For this review, take the finished solid that the model builds, in its own axes (mm). Face numbers are marked on the shaded views. A direction names the side the tool comes from. Coordinates: 2 decimals unless noted, no trailing zeros. Loops run counter-clockwise (first coordinate to the right, second up) from the corner with the lowest first, then second, coordinate; pieces in that order, holes last. Notation, with made-up numbers: (-0.5, 31.25) -> (49.5, 31.25) arc R20 cw to (49.5, 53.25) -> close; hole circle Ø11 at (-6, 89). An arc over 180 degrees is marked (long way). One line per item, written item: value.
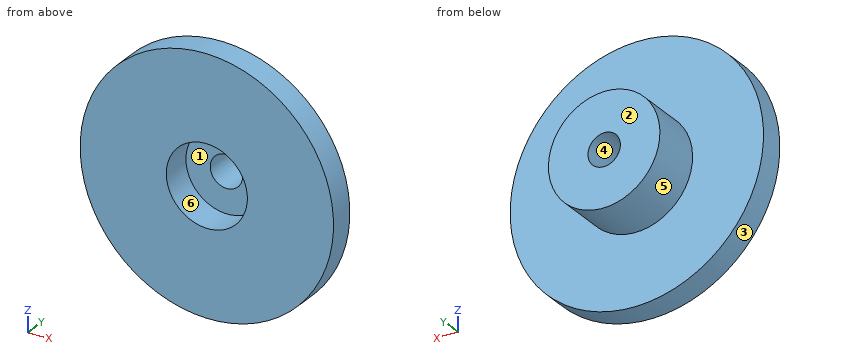
from build123d import *

# Parameters (mm, degrees)
SKETCH1_R           = 12.5
BOSS_EXTRUDE1_DEPTH = 2.5
SKETCH2_R           = 5.5
BOSS_EXTRUDE2_DEPTH = 5
HOLE1_D             = 3.2
HOLE1_DEPTH         = 100
HOLE1_CBORE_D       = 8
HOLE1_CBORE_DEPTH   = 3


with BuildPart() as part:
    # Sketch1 → Boss-Extrude1 (new body)
    with BuildSketch(Plane(origin=(0, 0, 0), x_dir=(1, 0, 0), z_dir=(0, 1, 0))):
        with Locations(Location((0, 0, 0), (0, 0, 270))):
            Circle(SKETCH1_R)
    extrude(amount=BOSS_EXTRUDE1_DEPTH)

    # Sketch2 → Boss-Extrude2 (add)
    with BuildSketch(Plane(origin=(0, 2.5, 0), x_dir=(1, 0, 0), z_dir=(0, 1, 0))):
        with Locations(Location((0, 0, 0), (0, 0, 270))):
            Circle(SKETCH2_R)
    extrude(amount=BOSS_EXTRUDE2_DEPTH)

    # Hole1
    with Locations(Plane(origin=(0, 0, 0), x_dir=(-1, 0, 0), z_dir=(0, -1, 0))):
        with Locations((0, 0)):
            CounterBoreHole(HOLE1_D / 2, HOLE1_CBORE_D / 2, HOLE1_CBORE_DEPTH, depth=HOLE1_DEPTH)


solid = part.part
1. For the marked faces 4, 5 and 6, list the 3-axis set-ups (+Z, -Z, +X, -X, +Y, -Y) from which the entire face can be reached by the end or side of a thin tool; tool diameter is ignored.
Return value:
face 4: +Y, -Y
face 5: +Y
face 6: -Y
2. To check wall thickness, follow probe 1 along X at (y, z) = (5.25, -0.25); probe 2 along Y at (x, z) = (-4.5, -9.5); probe 3 along Z at (x, y) = (1, 7.25). State the ranges of each line that lie inside material, in increasing order. Write a range as from..to.
Return value:
probe 1: x = -5.49..-1.58, 1.58..5.49
probe 2: y = 0..2.5
probe 3: z = -5.41..-1.25, 1.25..5.41
3. Take a section at C-C, the plane y = 4.5. Give the boundary of the cut face in (x, z), and give its area (3 significant figures).
Return value:
outline: circle Ø11 at (0, 0); hole circle Ø3.2 at (0, 0)
area: 87.0 mm2
4. Take a section at A-A, the plane z = 0. Give the boundary of the cut face in (x, y), and give its area (3 significant figures).
Return value:
outline: (-12.5, 0) -> (-4, 0) -> (-4, 3) -> (-1.6, 3) -> (-1.6, 7.5) -> (-5.5, 7.5) -> (-5.5, 2.5) -> (-12.5, 2.5) -> close; (1.6, 3) -> (4, 3) -> (4, 0) -> (12.5, 0) -> (12.5, 2.5) -> (5.5, 2.5) -> (5.5, 7.5) -> (1.6, 7.5) -> close
area: 79.1 mm2
5. The part is to be moulded in two halves that separate along X. For the marked faces 1, 2 and 3, say which applies: pulls with the +X half, pulls with the -X half, needs draft (parallel to the pull), parting line crosses it, or undercut.
Return value:
face 1: undercut
face 2: needs draft
face 3: parting line crosses it
6. Take a section at B-B, the plane x = 0. Give the boundary of the cut face in (y, z).
Return value:
outline: (0, -12.5) -> (2.5, -12.5) -> (2.5, -5.5) -> (7.5, -5.5) -> (7.5, -1.6) -> (3, -1.6) -> (3, -4) -> (0, -4) -> close; (0, 4) -> (3, 4) -> (3, 1.6) -> (7.5, 1.6) -> (7.5, 5.5) -> (2.5, 5.5) -> (2.5, 12.5) -> (0, 12.5) -> close
7. Insertion check: pin 1 Ø1 at (x, z) = (1.5, -1.5) entering from -Y; pin 2 Ø6 at (x, z) = (-6.5, -9.5) entering from +Y. Each pin has a flat end and moves straight along its axis. Give the tip position at first contact, or say it passes through.
Return value:
pin 1: stops at y = 3
pin 2: stops at y = 2.5
8. Take a section at D-D, the plane z = -10. Give the boundary of the cut face in (x, y), and give its area (3 significant figures).
Return value:
outline: (-7.5, 0) -> (7.5, 0) -> (7.5, 2.5) -> (-7.5, 2.5) -> close
area: 37.5 mm2
